Design review of the part built by this model. Coordinates are the model's own, in mm. A direction names the side the tool comes from. Give positions to 0.01 mm unless a question says otherwise; leave off trailing zeros. Write each loop counter-clockwise with the first axis right and the second up, starting at its lowest first coordinate (ties: lowest second). Pieces come first, ordered by that corner, then holes.
```python
from build123d import *

# Parameters (mm, degrees)
F0_R          = 10
F1_DEPTH      = 22
F1_DEPTH_BACK = 22
F2_DEPTH      = 8
F2_DEPTH_BACK = 8
F3_R          = 21.99999
F5_DEPTH      = 25


# Not quite as in the source:
# - a fillet or chamfer is up to 0.001 mm smaller than in the source, because OpenCascade refuses the exact size


with BuildPart() as f1:
    # F0 (on Front) → F1 (new body, two sides)
    with BuildSketch(Plane.XZ) as f1_sk:
        with BuildLine():
            Line((0, 40), (0, 16))
            Line((0, 16), (45.7235909998, 16))
            Line((45.7235909998, 16), (45.7235909998, 40))
            ThreePointArc((45.7235909998, 40), (22.8617954999, 62.8617954999), (0, 40))
        make_face()
        with Locations((22.8617954999, 40)):
            Circle(F0_R, mode=Mode.SUBTRACT)
        Polygon((0, 16), (0, 0), (118, 0), (118, 16), (45.7235909998, 16), align=None)
    extrude(amount=F1_DEPTH)
    extrude(f1_sk.sketch, amount=-F1_DEPTH_BACK)

    # F0 (on Front) → F2 (cut, two sides)
    with BuildSketch(Plane.XZ) as f2_sk:
        with BuildLine():
            Line((45.7235909998, 16), (118, 16))
            Line((118, 16), (118, 71.8919485807))
            Line((118, 71.8919485807), (0, 71.8919485807))
            Line((0, 71.8919485807), (0, 40))
            ThreePointArc((0, 40), (22.8617954999, 62.8617954999), (45.7235909998, 40))
            Line((45.7235909998, 40), (45.7235909998, 16))
        make_face()
        with BuildLine():
            Line((0, 40), (0, 16))
            Line((0, 16), (45.7235909998, 16))
            Line((45.7235909998, 16), (45.7235909998, 40))
            ThreePointArc((45.7235909998, 40), (22.8617954999, 62.8617954999), (0, 40))
        make_face()
        with Locations((22.8617954999, 40)):
            Circle(F0_R, mode=Mode.SUBTRACT)
    extrude(amount=-F2_DEPTH, mode=Mode.SUBTRACT)
    extrude(f2_sk.sketch, amount=F2_DEPTH_BACK, mode=Mode.SUBTRACT)

    # F3 (radius 22 in the source; OpenCascade refuses exactly that, so slightly less here)
    f3_edges = [f1.edges().sort_by_distance(p)[0] for p in [
        (118, -22, 8),
        (118, 22, 8),
    ]]
    fillet(f3_edges, radius=F3_R)

    # F4 (on face) → F5 (cut)
    with BuildSketch(Plane.XY.offset(16)):
        with BuildLine():
            ThreePointArc((70.8617954999, 8), (62.8617954999, 0), (70.8617954999, -8))
            Line((70.8617954999, -8), (94.8617954999, -8))
            ThreePointArc((94.8617954999, -8), (102.8617954999, 0), (94.8617954999, 8))
            Line((94.8617954999, 8), (70.8617954999, 8))
        make_face()
    extrude(amount=-F5_DEPTH, mode=Mode.SUBTRACT)


solid = f1.part
```
(1) Consider section B-B, the plane x = 74.5. Give the boundary of the cut face in (y, z), then the cut area to 3 significant figures.
Resolved:
outline: (-22, 0) - (-8, 0) - (-8, 16) - (-22, 16) - close; (8, 0) - (22, 0) - (22, 16) - (8, 16) - close
area: 448 mm2
(2) Clearance check with flat-ended pins moving along their axes: P1, Ø11, axis at y = 16, z = 32.5, coming from the +X side; P2, Ø12, axis at x = 71, y = 15, coming from the +Z side; P3, Ø8, axis at x = 38.5, y = 15.5, coming from the +Z side. State where each tip first meets the part, or that it passes through.
Resolved:
P1: stops at x = 45.72
P2: stops at z = 16
P3: stops at z = 59.68
(3) Tool access review of faces 1 (the face through (23, 8, 29)), 2 (the face through (58, 0, 16)), 3 (the face through (83, -8, 8)), 4 (the face through (45.724, 15, 28)): name each direction out of +Z, -Z, +X, -X, +Y, -Y from which nothing blocks a thin tool from reaching the whole face with its end or side.
Resolved:
face 1: +Z, +X, -X
face 2: +Z, +X
face 3: +Z, -Z
face 4: +Z, +X, +Y, -Y
(4) Mouldability with a two-part tool opening along X and no side actions: class faces 5 (the face through (102.86, -0.18, 8.11)), 6 (the face through (111.73, 15.38, 8.11)), 7 (the face through (23, -8, 29)) as pulls with the +X half, pulls with the -X half, needs draft (parallel to the pull), parting line crosses it, or undercut.
Resolved:
face 5: undercut
face 6: pulls with the +X half
face 7: needs draft
(5) Consider section A-A, the plane z = 24. Give the boundary of the cut face in (x, y), then the cut area to 3 significant figures.
Resolved:
outline: (0, -22) - (45.72, -22) - (45.72, -8) - (0, -8) - close; (0, 8) - (45.72, 8) - (45.72, 22) - (0, 22) - close
area: 1,280 mm2
(6) To check wall thickness, follow L1, parallel to Y at x = 45, z = 31.5; L2, parallel to Z at x = 7, y = 1; L3, parallel to X at y = -15, z = 32.5. State the ranges of each line that lie inside material, in increasing order.
Resolved:
L1: y = -22 to -8, 8 to 22
L2: z = 0 to 16
L3: x = 0 to 16.25, 29.48 to 45.72
(7) Consider section C-C, the plane y = 17.5. Give the boundary of the cut face in (x, z).
Resolved:
outline: (0, 0) - (109.33, 0) - (109.33, 16) - (45.72, 16) - (45.72, 40) arc R22.86 ccw to (0, 40) - close; hole circle Ø20 at (22.86, 40)
